Check sheet for the modelled part. Datum: model origin and axes. Units: mm. Face numbers are marked on the shaded views. A direction names the side the tool comes from. Round coordinates to 2 decimals unless told otherwise and drop trailing zeros. Write each loop counter-clockwise with the first axis right and the second up, starting at its lowest first coordinate (ties: lowest second). Pieces come first, ordered by that corner, then holes. Notation, with made-up numbers: (59, 69.5) -> (87, 69.5) arc R26 cw to (87, 93.5) -> close; hole circle Ø2 at (85.5, -19). An arc over 180 degrees is marked (long way). One line per item, written item: value.
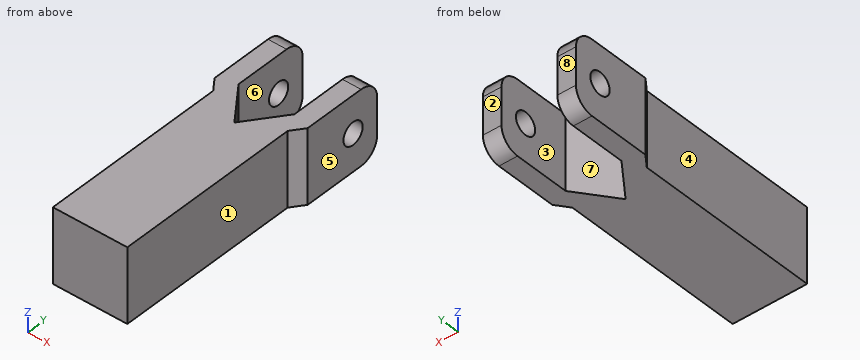
from build123d import *

# Parameters (mm, degrees)
ESTRUSIONE_ESTRUSIONE1_DEPTH = 20
SCHIZZO2_R                   = 6
TAGLIO_ESTRUSIONE1_DEPTH     = 40
RACCORDO1_R                  = 10


with BuildPart() as part:
    # Schizzo1 → Estrusione-Estrusione1 (new, symmetric)
    with BuildSketch(Plane.XY):
        Polygon((-25, 150), (-25, 106.666666667), (-20, 100), (-20, 0), (0, 0), (0, 90), (-15, 110), (-15, 150), align=None)
    extrude(amount=ESTRUSIONE_ESTRUSIONE1_DEPTH, both=True)

    # Schizzo2 → Taglio-Estrusione1 (cut)
    with BuildSketch(Plane.ZY.offset(25)):
        with Locations(Location((0, 135, 0), (0, 0, 270))):
            Circle(SCHIZZO2_R)
    extrude(amount=-TAGLIO_ESTRUSIONE1_DEPTH, mode=Mode.SUBTRACT)

    # Specchia1: part across plane


with BuildPart() as part_1:
    add(part.part)
    add(part.part.mirror(Plane(origin=(0, 0, 20), x_dir=(0, 0, 1), z_dir=(-1, 0, 0))))

    # Raccordo1
    raccordo1_edges = [part_1.edges().sort_by_distance(p)[0] for p in [
        (-20, 150, -20),
        (20, 150, 20),
        (20, 150, -20),
        (-20, 150, 20),
    ]]
    fillet(raccordo1_edges, radius=RACCORDO1_R)


solid = part_1.part
Item 1: Depth check by flat-ended pin: pin 1 (12 mm diameter, centred on y = 30.5, z = -4.5, fed in from -X); pin 2 (1 mm diameter, centred on x = 6, z = 9, fed in from +Y); pin 3 (5 mm diameter, centred on y = 69.5, z = 11, fed in from +X). Enter the tip coordinate at first touch or a pass-through.
Result set:
pin 1: x = -20
pin 2: y = 98.67
pin 3: x = 20
Item 2: Release check for a two-part mould opening along X. For the marked faces 5, 6, 7 and 8 record: pulls with the +X half, pulls with the -X half, needs draft (parallel to the pull), parting line crosses it, or undercut.
Result set:
face 5: pulls with the +X half
face 6: undercut
face 7: undercut
face 8: needs draft
Item 3: Sectioned sample at D-D (y = 40). Enter the section's corners in (x, z), then the cut area to 3 significant figures.
Result set:
outline: (-20, -20) -> (20, -20) -> (20, 20) -> (-20, 20) -> close
area: 1,600 mm^2
Item 4: Material ranges on line 1 along Z through (x, y) = (-21, 135); line 2 along X through (y, z) = (140, -5); line 3 along X through (y, z) = (8, -6), recorded low to high.
Result set:
line 1: -20 to -6, 6 to 20
line 2: -25 to -15, 15 to 25
line 3: -20 to 20
Item 5: Tool access check on the marked faces 1, 2, 3 and 4. Record the directions out of +Z, -Z, +X, -X, +Y, -Y that give a thin tool (end or side, any length) a straight path to the whole face; none if there is none.
Result set:
face 1: +Z, -Z, +X, -Y
face 2: +Z, -Z, +X, -X, +Y
face 3: +Z, -Z, +Y
face 4: +Z, -Z, -X, -Y
Item 6: Sectioned sample at C-C (x = 16.5). Enter the section's corners in (y, z).
Result set:
outline: (0, -20) -> (140, -20) arc R10 ccw to (150, -10) -> (150, 10) arc R10 ccw to (140, 20) -> (0, 20) -> close; hole circle Ø12 at (135, 0)
Item 7: Sectioned sample at B-B (z = 0). Enter the section's corners in (x, y).
Result set:
outline: (-25, 106.67) -> (-20, 100) -> (-20, 0) -> (20, 0) -> (20, 100) -> (25, 106.67) -> (25, 129) -> (15, 129) -> (15, 110) -> (0, 90) -> (-15, 110) -> (-15, 129) -> (-25, 129) -> close; (-25, 141) -> (-15, 141) -> (-15, 150) -> (-25, 150) -> close; (15, 141) -> (25, 141) -> (25, 150) -> (15, 150) -> close
Item 8: Sectioned sample at A-A (y = 135). Enter the section's corners in (x, z), then the cut area to 3 significant figures.
Result set:
outline: (-25, -20) -> (-15, -20) -> (-15, -6) -> (-25, -6) -> close; (-25, 6) -> (-15, 6) -> (-15, 20) -> (-25, 20) -> close; (15, -20) -> (25, -20) -> (25, -6) -> (15, -6) -> close; (15, 6) -> (25, 6) -> (25, 20) -> (15, 20) -> close
area: 560 mm^2
